The listing builds one solid part. Answer for the finished solid, in the listing's coordinates (mm). Face numbers are marked on the shaded views. A direction names the side the tool comes from. Give positions to 0.01 mm unless a question says otherwise; leave off trailing zeros. Order: outer loops, then holes, each group sorted by start corner. A loop starts at its lowest first (then second) coordinate and runs counter-clockwise, first axis right, second up. Notation, with made-up numbers: (17.5, 78) - (51.5, 78) arc R18 cw to (51.5, 113) - close; hole circle Ø2 at (86, 21.5). An arc over 180 degrees is marked (long way). Answer in a Markdown table with one row per item.
from build123d import *

# Parameters (mm, degrees)
BOSS_EXTRUDE1_DEPTH = 12.7
BOSS_EXTRUDE2_DEPTH = 6.805909
SKETCH3_R           = 2.159
CUT_EXTRUDE1_DEPTH  = 155.273638788
SKETCH5_R           = 2.159
CUT_EXTRUDE2_DEPTH  = 6.805909488
FILLET1_R           = 3.175
SKETCH6_R           = 12.7
BOSS_EXTRUDE3_DEPTH = 3.175
FILLET2_R           = 10.16


with BuildPart() as part:
    # Sketch1 → Boss-Extrude1 (new body)
    with BuildSketch(Plane(origin=(0, 0, 0), x_dir=(1, 0, 0), z_dir=(0, 1, 0))):
        Polygon((0, 25.4), (38.1, 25.4), (101.6, 25.4), (101.6, 18.594090512), (38.1, -25.4), (0, -25.4), align=None)
    extrude(amount=BOSS_EXTRUDE1_DEPTH)

    # Sketch2 → Boss-Extrude2 (add)
    with BuildSketch(Plane(origin=(0, 0, -25.4), x_dir=(-1, 0, 0), z_dir=(0, 0, -1))):
        Polygon((-63.5, 19.133437227), (-63.5, -6.433437227), (-76.283437227, -28.575), (-126.916562773, -28.575), (-139.7, -6.433437227), (-139.7, 19.133437227), (-126.916562773, 41.275), (-76.283437227, 41.275), align=None)
    extrude(amount=-BOSS_EXTRUDE2_DEPTH)

    # Sketch3 → Cut-Extrude1 (cut, through all)
    with BuildSketch(Plane(origin=(0, 0, -25.4), x_dir=(-1, 0, 0), z_dir=(0, 0, -1))):
        with Locations((-88.9, 25.4)):
            Circle(SKETCH3_R)
        with Locations((-88.9, -12.7)):
            Circle(SKETCH3_R)
    extrude(amount=-CUT_EXTRUDE1_DEPTH, mode=Mode.SUBTRACT)

    # Sketch5 → Cut-Extrude2 (cut)
    with BuildSketch(Plane(origin=(0, 0, -25.4), x_dir=(-1, 0, 0), z_dir=(0, 0, -1))):
        with Locations((-114.3, 0)):
            Circle(SKETCH5_R)
        with Locations((-114.3, 12.7)):
            Circle(SKETCH5_R)
    extrude(amount=-CUT_EXTRUDE2_DEPTH, mode=Mode.SUBTRACT)

    # Fillet1
    fillet1_edges = [part.edges().sort_by_distance(p)[0] for p in [
        (101.6, 6.35, -18.594090512),
        (31.75, 0, -25.4),
        (82.55, 0, -18.594091),
        (31.75, 12.7, -25.4),
        (82.55, 12.7, -18.594091),
    ]]
    fillet(fillet1_edges, radius=FILLET1_R)

    # Sketch6 → Boss-Extrude3 (add)
    with BuildSketch(Plane(origin=(0, 12.7, 0), x_dir=(1, 0, 0), z_dir=(0, 1, 0))):
        with Locations(Location((19.05, 0, 0), (0, 0, 270))):
            Circle(SKETCH6_R)
    extrude(amount=BOSS_EXTRUDE3_DEPTH)

    # Fillet2
    fillet2_edges = [part.edges().sort_by_distance(p)[0] for p in [
        (38.1, 6.35, 25.4),
        (0, 6.35, 25.4),
    ]]
    fillet(fillet2_edges, radius=FILLET2_R)


solid = part.part
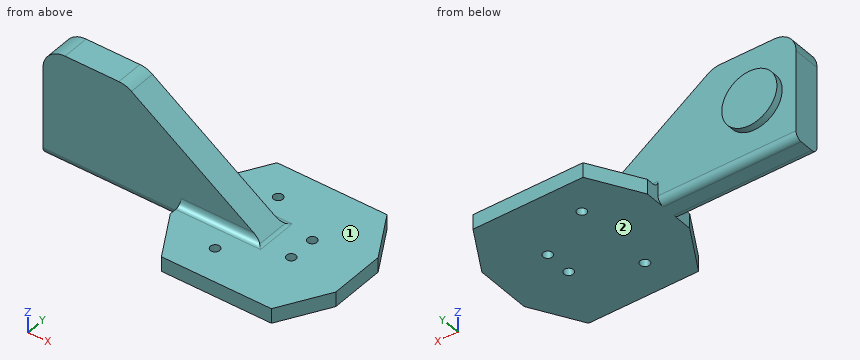
Item 1: Each of these flat-tipped pins is pushed along its axis until it touches: P1, Ø7.5, axis at x = 25, z = 0.5, coming from the +Y side (3 decimals); P2, Ø12, axis at y = 11.5, z = 16, coming from the +X side; P3, Ø5, axis at y = 15.5, z = -20.5, coming from the -X side; P4, Ø3, axis at x = 44.5, y = 3, coming from the -Z side. Where does it stop, or does it pass through?
Answer block:
| item | result |
|---|---|
| P1 | y = 15.875 |
| P2 | x = 60.33 |
| P3 | x = 63.5 |
| P4 | z = -25.4 |
Item 2: Find section C-C on x = 19.05. Write down the section's boundary in (y, z) (3 decimals).
Answer block:
| item | result |
|---|---|
| outline | (0, -22.225) arc R3.175 ccw to (3.175, -25.4) - (9.525, -25.4) arc R3.175 ccw to (12.7, -22.225) - (12.7, -12.7) - (15.875, -12.7) - (15.875, 12.7) - (12.7, 12.7) - (12.7, 25.4) - (0, 25.4) - close |
Item 3: Consider line 1 (Y direction, x = 114, z = -22) (3 decimals); line 2 (Y direction, x = 88.9, z = -20.25) (3 decimals); line 3 (Z direction, x = 113.5, y = -12). Determine where each line is inside the solid, lowest interval first.
Answer block:
| item | result |
|---|---|
| line 1 | -28.575 to -2.138, 2.138 to 10.562, 14.838 to 41.275 |
| line 2 | -28.575 to -14.859, -10.541 to 23.241, 27.559 to 41.275 |
| line 3 | -25.4 to -18.59 |
Item 4: Find section D-D on y = 5.5. Write down the section's boundary in (x, z) (3 decimals).
Answer block:
| item | result |
|---|---|
| outline | (0, -25.4) - (139.7, -25.4) - (139.7, -18.594) - (102.592, -18.594) arc R3.175 cw to (100.784, -18.029) - (40.71, 23.591) arc R10.16 ccw to (34.924, 25.4) - (10.16, 25.4) arc R10.16 ccw to (0, 15.24) - close |
Item 5: Find section B-B on y = 25.4. Write down the section's boundary in (x, z).
Answer block:
| item | result |
|---|---|
| outline | (67.12, -25.4) - (86.74, -25.4) - (86.74, -18.59) - (67.12, -18.59) - close; (91.06, -25.4) - (136.08, -25.4) - (136.08, -18.59) - (91.06, -18.59) - close |
Item 6: Find section A-A on x = 114.3. Write down the section's boundary in (y, z) (3 decimals).
Answer block:
| item | result |
|---|---|
| outline | (-28.575, -25.4) - (-2.159, -25.4) - (-2.159, -18.594) - (-28.575, -18.594) - close; (2.159, -25.4) - (10.541, -25.4) - (10.541, -18.594) - (2.159, -18.594) - close; (14.859, -25.4) - (41.275, -25.4) - (41.275, -18.594) - (14.859, -18.594) - close |
Item 7: Which of the six approach directions +Z, -Z, +X, -X, +Y, -Y give full straight-line access (tool end or side, diameter ignored) to the marked faces 1 and 2?
Answer block:
| item | result |
|---|---|
| face 1 | +Z, +X |
| face 2 | -Z, +X, -X, +Y, -Y |
